```python
from build123d import *

# Parameters (mm, degrees)
SKETCH_1_R          = 1.4
EXTRUDE_1_DEPTH     = 3
SKETCH_2_R          = 4
EXTRUDE_3_DEPTH     = 210
SKETCH_3_W          = 8
SKETCH_3_H          = 5.7
EXTRUDE_4_DEPTH     = 3
CUT_EXTRUDE_1_DEPTH = 214.705779051


with BuildPart() as part:
    # 草图1 → 凸台-拉伸1 (new body)
    with BuildSketch(Plane.XY):
        with BuildLine():
            Line((-4, -11.4), (-4, 11.4))
            ThreePointArc((-4, 11.4), (0, 15.4), (4, 11.4))
            Line((4, 11.4), (4, -11.4))
            ThreePointArc((4, -11.4), (0, -15.4), (-4, -11.4))
        make_face()
        with Locations((0, 11.4)):
            Circle(SKETCH_1_R, mode=Mode.SUBTRACT)
        with Locations(Location((0, -11.4, 0), (0, 0, 180))):
            Circle(SKETCH_1_R, mode=Mode.SUBTRACT)
    extrude(amount=EXTRUDE_1_DEPTH)

    # 草图2 → 凸台-拉伸3 (add)
    with BuildSketch(Plane.XY.offset(3)):
        Circle(SKETCH_2_R)
    extrude(amount=EXTRUDE_3_DEPTH)

    # 草图3 → 凸台-拉伸4 (add)
    with BuildSketch(Plane(origin=(0, 0, 0), x_dir=(-1, 0, 0), z_dir=(0, 0, -1))):
        with Locations((0, 2.85)):
            Rectangle(SKETCH_3_W, SKETCH_3_H)
        with Locations((0, -2.85)):
            Rectangle(SKETCH_3_W, SKETCH_3_H)
    extrude(amount=EXTRUDE_4_DEPTH)

    # 草图5 → 切除-拉伸1 (cut, through all)
    with BuildSketch(Plane(origin=(4, 0, 0), x_dir=(0, 0, -1), z_dir=(1, 0, 0))):
        Polygon((0, 5.7), (3, 0), (3, 5.7), align=None)
        Polygon((3, -5.7), (3, 0), (0, -5.7), align=None)
    extrude(amount=-CUT_EXTRUDE_1_DEPTH, mode=Mode.SUBTRACT)


solid = part.part
```
Verification items for the finished model (mm, model axes). A direction names the side the tool comes from. Round coordinates to 2 decimals unless told otherwise and drop trailing zeros. Write each loop counter-clockwise with the first axis right and the second up, starting at its lowest first coordinate (ties: lowest second). Pieces come first, ordered by that corner, then holes. Notation, with made-up numbers: (77.25, -4) - (101.25, -4) arc R29 cw to (101.25, 18) - close; hole circle Ø9 at (25, 54). An arc over 180 degrees is marked (long way). Answer as a JSON object with one key per item and string values. Group by question number.
Q1. Go/stop test with flat-tipped pins: pin 1 Ø4 at (x, y) = (2.5, -8) entering from +Z; pin 2 Ø1.5 at (x, z) = (-1.5, 110.5) entering from -Y; pin 3 Ø2.5 at (x, y) = (0, 11.4) entering from +Z; pin 4 Ø1.5 at (x, z) = (-3, 85.5) entering from -Y. Record where each tip stops, or that it passes through.
Q2. Section check A-A, the plane x = 0. Enter the section's corners in (y, z), plus the area to 3 significant figures.
Q3. Thickness scan on line 1 (Y direction, x = 0, z = 1.6); line 2 (X direction, y = -11.4, z = 1.4); line 3 (Z direction, x = -0.75, y = 8.5). Record the ranges inside material, lowest first.
Q4. Section check B-B, the plane z = 98. Enter the section's corners in (x, y), plus the area to 3 significant figures.
Q5. Tool access check on faces 1 (the flat face through (0, -9, 0)), 2 (the cylindrical face through (-0.867, -3.905, 106.53)), 3 (the flat face through (0.1, 9.5, 0)), 4 (the flat face through (0, 0, 213)). Record the directions out of +Z, -Z, +X, -X, +Y, -Y that give a thin tool (end or side, any length) a straight path to the whole face; none if there is none.
Found:
{
 "1": {"pin 1": "stops at z = 3", "pin 2": "stops at y = -3.93", "pin 3": "passes through", "pin 4": "stops at y = -3.31"},
 "2": {"outline": "(-15.4, 0) - (-12.8, 0) - (-12.8, 3) - (-15.4, 3) - close; (-10, 0) - (-5.7, 0) - (0, -3) - (5.7, 0) - (10, 0) - (10, 3) - (4, 3) - (4, 213) - (-4, 213) - (-4, 3) - (-10, 3) - close; (12.8, 0) - (15.4, 0) - (15.4, 3) - (12.8, 3) - close", "area": "1,770 mm^2"},
 "3": {"line 1": "y = -15.4 to -12.8, -10 to 10, 12.8 to 15.4", "line 2": "x = -4 to -1.4, 1.4 to 4", "line 3": "z = 0 to 3"},
 "4": {"outline": "circle Ø8 at (0, 0)", "area": "50.3 mm^2"},
 "5": {"face 1": "-Z, +X, -X, -Y", "face 2": "+Z", "face 3": "-Z, +X, -X, +Y", "face 4": "+Z, +X, -X, +Y, -Y"}
}
